```python
from build123d import *

# Parameters (mm, degrees)
PAD007_DEPTH         = 350
POCKET009_DEPTH      = 2.001
POCKET009_DEPTH_BACK = 20.001
PAD008_DEPTH         = 20
SKETCH023_R          = 1.5
SKETCH023_R_2        = 1.21447
POCKET010_DEPTH      = 3
SKETCH024_R          = 1.5
POCKET011_DEPTH      = 5
SKETCH025_R          = 1.5
POCKET012_DEPTH      = 5
SKETCH026_R          = 1.5
POCKET013_DEPTH      = 5
SKETCH070_R          = 1.5
POCKET046_DEPTH      = 5


with BuildPart() as part:
    # Sketch020 (on Face1 of Binder004) → Pad007 (new body)
    with BuildSketch(Plane(origin=(0, -4.1, 0), x_dir=(-1, 0, 0), z_dir=(0, 1, 0))):
        Polygon((-1160, -341.2), (-1160, 106.0068995871), (-1180, 103.0899380794), (-1180, 105.0899380794), (-1158, 108.0068995871), (-1158, -343.2), (-1160, -343.2), (-1180, -343.2), (-1180, -341.2), align=None)
    extrude(amount=PAD007_DEPTH)

    # Sketch021 (on Face3 of Pad007) → Pocket009 (cut, two sides)
    with BuildSketch(Plane.YZ.offset(1160)) as pocket009_sk:
        Polygon((-4.1, -203.2), (175.5753880751, 108.0069), (-4.1, 108.0069), align=None)
    extrude(amount=-POCKET009_DEPTH, mode=Mode.SUBTRACT)
    extrude(pocket009_sk.sketch, amount=POCKET009_DEPTH_BACK, mode=Mode.SUBTRACT)

    # Sketch022 (on Face7 of Pocket009) → Pad008 (join)
    with BuildSketch(Plane.YZ.offset(1160)):
        Polygon((-4.1, -341.2), (-2.1, -341.2), (-2.1, -203.2), (174.7363949149, 103.0899380794), (172.7363949149, 103.0899380794), (-4.1, -203.2), align=None)
    extrude(amount=PAD008_DEPTH)

    # Sketch023 (on Face1 of Binder004) → Pocket010 (cut)
    with BuildSketch(Plane(origin=(0, -4.1, 0), x_dir=(-1, 0, 0), z_dir=(0, 1, 0))):
        with Locations((-1170, -333.2)):
            Circle(SKETCH023_R)
        with Locations((-1168.78553, -273.2)):
            Circle(SKETCH023_R_2)
        with Locations((-1170, -213.2)):
            Circle(SKETCH023_R)
    extrude(amount=POCKET010_DEPTH, mode=Mode.SUBTRACT)

    # Sketch024 (on Face11 of Pocket010) → Pocket011 (cut)
    with BuildSketch(Plane(origin=(0, 84.9131338325, -49.0245698635), x_dir=(1, 0, 0), z_dir=(0, -0.8660256282, 0.4999996113))):
        with Locations((1170, -168.059563)):
            Circle(SKETCH024_R)
        with Locations((1170, -2.4571175269)):
            Circle(SKETCH024_R)
        with Locations((1170, 165.290966)):
            Circle(SKETCH024_R)
        with Locations((1170, -108.059563)):
            Circle(SKETCH024_R)
        with Locations((1170, -51.413154)):
            Circle(SKETCH024_R)
        with Locations((1170, 46.410008)):
            Circle(SKETCH024_R)
        with Locations((1170, 103.145328)):
            Circle(SKETCH024_R)
    extrude(amount=-POCKET011_DEPTH, mode=Mode.SUBTRACT)

    # Sketch025 (on Face10 of Pocket011) → Pocket012 (cut)
    with BuildSketch(Plane(origin=(34.0789471152, 0, 257.0266472675), x_dir=(0.9913242799, 0, -0.131438853), z_dir=(0.131438853, 0, 0.9913242799))):
        with Locations((1145.949749, 183.891094)):
            Circle(SKETCH025_R)
        with Locations((1145.949749, 259.895547)):
            Circle(SKETCH025_R)
        with Locations((1145.949749, 335.9)):
            Circle(SKETCH025_R)
    extrude(amount=-POCKET012_DEPTH, mode=Mode.SUBTRACT)

    # Sketch026 (on Face6 of Pocket012) → Pocket013 (cut)
    with BuildSketch(Plane.XY.offset(-341.2)):
        with Locations((1170, 335.9)):
            Circle(SKETCH026_R)
        with Locations((1170, 258.9)):
            Circle(SKETCH026_R)
        with Locations((1170, 171.9)):
            Circle(SKETCH026_R)
        with Locations((1170, 89.9)):
            Circle(SKETCH026_R)
        with Locations((1170, 7.9)):
            Circle(SKETCH026_R)
    extrude(amount=-POCKET013_DEPTH, mode=Mode.SUBTRACT)

    # Sketch070 (on Face1 of Binder020) → Pocket046 (cut)
    with BuildSketch(Plane(origin=(1156, 0, 0), x_dir=(0, -1, 0), z_dir=(-1, 0, 0))):
        with Locations((-7.917049, -213.170471)):
            Circle(SKETCH070_R)
        with Locations((-89.912786, -213.170471)):
            Circle(SKETCH070_R)
        with Locations((-171.908524, -213.170471)):
            Circle(SKETCH070_R)
        with Locations((-253.904262, -213.170471)):
            Circle(SKETCH070_R)
        with Locations((-335.9, -213.170471)):
            Circle(SKETCH070_R)
    extrude(amount=-POCKET046_DEPTH, mode=Mode.SUBTRACT)


with BuildPart() as part_1:
    # Body004 placement: moved
    add(part.part.moved(Location((-280, 4, 0))))


solid = part_1.part
```
CAD build for the part. Positions are in the model's coordinates, mm. A direction names the side the tool comes from. Coordinates: 2 decimals unless noted, no trailing zeros. Write each loop counter-clockwise with the first axis right and the second up, starting at its lowest first coordinate (ties: lowest second). Pieces come first, ordered by that corner, then holes.
(1) Drill centre lines: probe 1 along Y at (x, z) = (890, -342.3); probe 2 along X at (y, z) = (0.9, -333.2); probe 3 along Z at (x, y) = (894.75, 304.5). Where is each one in solid material? Low to high.
(2) Flat gauge pins, fed straight in: pin 1 (5 mm diameter, centred on x = 890, y = 339.9, fed in from +Z); pin 2 (2.5 mm diameter, centred on y = 339.9, z = -213.17, fed in from +X); pin 3 (5 mm diameter, centred on x = 883.5, z = -98, fed in from +Y); pin 4 (8 mm diameter, centred on x = 888.5, y = 147, fed in from +Z). Where does each tip first touch, or does it go through?
(3) Two-plate mould, pull along Z, no slides. Class faces 1 (the face through (880, 212, -170)), 2 (the face through (878.46, 89.32, -48.32)), 3 (the face through (878, 211, -165)): +Z half, -Z half, draft (parallel to the pull), parting line (faces both ways), or undercut.
(4) Cut at B-B, the plane z = -250. List the corners of the cut face in (x, y).
(5) 3-axis set-ups, long thin cutter, end or side, ignore diameter. For faces 4 (the face through (887.64, 89.08, -52.2)), 5 (the face through (891, -0.1, -272)): which of +Z, -Z, +X, -X, +Y, -Y reach the whole face in a straight line?
(6) Cut at A-A, the plane y = 204. List the corners of the cut face in (x, z), and give its area (3 significant figures).
Geometry says:
1. probe 1: y = -0.1 to 10.4, 13.4 to 92.4, 95.4 to 174.4, 177.4 to 261.4, 264.4 to 338.4, 341.4 to 349.9
1. probe 2: x = 878 to 888.5, 891.5 to 900
1. probe 3: z = -343.2 to -341.2, 103.86 to 105.79
2. pin 1: stops at z = 106.75
2. pin 2: passes through
2. pin 3: stops at y = 64.08
2. pin 4: stops at z = 58.51
3. face 1: undercut
3. face 2: +Z half
3. face 3: draft
4. outline: (878, -0.1) - (900, -0.1) - (900, 1.9) - (880, 1.9) - (880, 349.9) - (878, 349.9) - close
5. face 4: +X, +Y
5. face 5: +Z, -Z, +X, -X, -Y
6. outline: (878, -343.2) - (900, -343.2) - (900, -341.2) - (880, -341.2) - (880, 106.01) - (900, 103.09) - (900, 105.09) - (878, 108.01) - close
6. area: 979 mm2
